```python
from build123d import *

# Parameters (mm, degrees)
SKETCH1_W                  = 38.1
SKETCH1_H                  = 41.275
SKETCH1_R                  = 5.55625
BOSS_EXTRUDE1_DEPTH        = 12.7
F_10_32_TAPPED_HOLE1_D     = 4.0386
F_10_32_TAPPED_HOLE1_DEPTH = 15.875
F_10_32_TAPPED_HOLE1_TIP   = 1.213317848


with BuildPart() as part:
    # Sketch1 → Boss-Extrude1 (new body)
    with BuildSketch(Plane.XY):
        with Locations((0, 20.6375)):
            Rectangle(SKETCH1_W, SKETCH1_H)
        with Locations((0, 28.575)):
            Circle(SKETCH1_R, mode=Mode.SUBTRACT)
    extrude(amount=BOSS_EXTRUDE1_DEPTH)

    # #10-32 Tapped Hole1
    with Locations(Plane(origin=(0, 0, 0), x_dir=(-1, 0, 0), z_dir=(0, -1, 0))):
        with Locations((-13.97, -6.35), (13.97, -6.35)):
            Hole(F_10_32_TAPPED_HOLE1_D / 2, depth=F_10_32_TAPPED_HOLE1_DEPTH)
            with Locations((0, 0, -(F_10_32_TAPPED_HOLE1_DEPTH + F_10_32_TAPPED_HOLE1_TIP / 2))):  # 118° drill point
                Cone(0, F_10_32_TAPPED_HOLE1_D / 2, F_10_32_TAPPED_HOLE1_TIP, mode=Mode.SUBTRACT)


solid = part.part
```
Geometry: final body of the model. Coordinates: model frame, mm. A direction names the side the tool comes from. Round coordinates to 2 decimals unless told otherwise and drop trailing zeros. Write each loop counter-clockwise with the first axis right and the second up, starting at its lowest first coordinate (ties: lowest second). Pieces come first, ordered by that corner, then holes. Notation, with made-up numbers: (-31, -21) -> (-19, -21) arc R17 ccw to (-19, -16) -> close; hole circle Ø2 at (50, 38). An arc over 180 degrees is marked (long way). Return JSON: item names as keys, results as strings.
Q1. Section B-B on x = 0. Return the cut outline in (y, z) (3 decimals), and give its area (3 significant figures).
From the geometry:
{"outline": "(0, 0) -> (23.019, 0) -> (23.019, 12.7) -> (0, 12.7) -> close; (34.131, 0) -> (41.275, 0) -> (41.275, 12.7) -> (34.131, 12.7) -> close", "area": "383 mm2"}
Q2. Ray query, line 1 (Y direction, x = -1, z = 5.25) (3 decimals); line 2 (Y direction, x = -0.5, z = 4.75) (3 decimals); line 3 (X direction, y = 28.5, z = 1.75). Return the intervals inside material, ascending.
From the geometry:
{"line 1": "0 to 23.109, 34.041 to 41.275", "line 2": "0 to 23.041, 34.109 to 41.275", "line 3": "-19.05 to -5.56, 5.56 to 19.05"}
Q3. Section C-C on y = 32.5. Return the cut outline in (x, z).
From the geometry:
{"outline": "(-19.05, 0) -> (-3.93, 0) -> (-3.93, 12.7) -> (-19.05, 12.7) -> close; (3.93, 0) -> (19.05, 0) -> (19.05, 12.7) -> (3.93, 12.7) -> close"}
Q4. Section A-A on y = 14. Return the cut outline in (x, z).
From the geometry:
{"outline": "(-19.05, 0) -> (19.05, 0) -> (19.05, 12.7) -> (-19.05, 12.7) -> close; hole circle Ø4.04 at (-13.97, 6.35); hole circle Ø4.04 at (13.97, 6.35)"}
Q5. First-contact query: pin 1 Ø4.5 at (x, z) = (-13.97, 6.35) entering from -Y; pin 2 Ø3 at (x, z) = (13.97, 6.35) entering from -Y. Flat tips, straight axial feed; report the tip coordinate or a pass-through.
From the geometry:
{"pin 1": "y = 0", "pin 2": "y = 16.19"}
Q6. Set-up query: faces 4 (the flat face through (-19.05, 20, 6)), 5 (the cylindrical face through (-15.987, 8.049, 6.261)). Return all of +Z, -Z, +X, -X, +Y, -Y with unobstructed straight access to the full face (end or side cutting, diameter ignored); none if empty.
From the geometry:
{"face 4": "+Z, -Z, -X, +Y, -Y", "face 5": "-Y"}
Q7. Mould query, pull axis Y, two halves, no side actions, for faces 1 (the cylindrical face through (-4.095, 32.33, 6.261)), 2 (the flat face through (0, 41.275, 6)), 3 (the flat face through (19.05, 20, 6)). Classes: +Y half, -Y half, draft (parallel to the pull), parting line (faces both ways), or undercut.
From the geometry:
{"face 1": "undercut", "face 2": "+Y half", "face 3": "draft"}
